Here's the drawing with two shaded views (mm, measured from the low corner). I have some questions. Give positions to 0.01 mm unless a question says otherwise; leave off trailing zeros. Loops run counter-clockwise (first coordinate to the right, second up) from the corner with the lowest first, then second, coordinate; pieces in that order, holes last. Notation, with made-up numbers: M -21,-32.75 L 3,-32.75 A32 cw 3,-1.75 Z; hole C 8,-35.5 d5. An arc over 180 degrees is marked long. Write item = value, one per line. Start each with the question number.
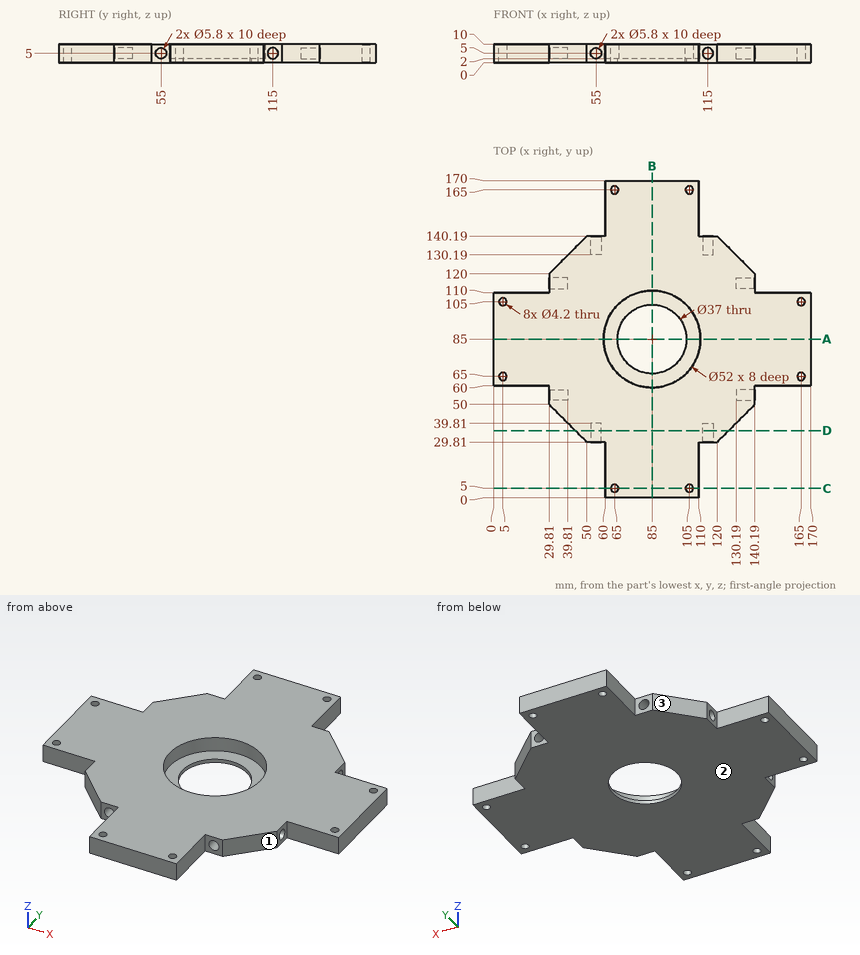
Q1. Will these pins go through, and if not, where does the flat tip stop? pin 1 (1.7 mm diameter, centred on y = 55.5, z = 6, fed in from -X); pin 2 (5 mm diameter, centred on x = 115, z = 5, fed in from +Y); pin 3 (2 mm diameter, centred on y = 19.5, z = 5.5, fed in from +X).
Q2. If we section it at A-A, the plane y = 85: List the corners of the cut face in (x, z) for me.
Q3. If we section it at C-C, the plane y = 5: List the corners of the cut face in (x, z) for me, then the cut area to 3 significant figures.
Q4. If I drill on line 1 along X through (y, z) = (165, 3); line 2 along X through (y, z) = (33.5, 5); line 3 along X through (y, z) = (104, 5.5), over which ranges is the centre line in solid material (lowest first)?
Q5. We'd pull the mould along Y, two halves only. Please class the marked faces 1, 2 and 3: pulls with the +Y half, pulls with the -Y half, needs draft (parallel to the pull), parting line crosses it, or undercut.
Q6. If we section it at D-D, the plane y = 36: List the corners of the cut face in (x, z) for me.
Resolved:
q1.pin_1 = 39.81
q1.pin_2 = 130.19
q1.pin_3 = 110
q2.outline = M 0,0 L 66.5,0 L 66.5,2 L 59,2 L 59,10 L 0,10 Z; M 103.5,0 L 170,0 L 170,10 L 111,10 L 111,2 L 103.5,2 Z
q3.outline = M 60,0 L 62.9,0 L 62.9,10 L 60,10 Z; M 67.1,0 L 102.9,0 L 102.9,10 L 67.1,10 Z; M 107.1,0 L 110,0 L 110,10 L 107.1,10 Z
q3.area = 416 mm²
q4.line_1 = 60 to 62.9, 67.1 to 102.9, 107.1 to 110
q4.line_2 = 46.31 to 52.1, 57.9 to 112.1, 117.9 to 123.69
q4.line_3 = 0 to 3.15, 6.85 to 67.25, 102.75 to 163.15, 166.85 to 170
q5.face_1 = pulls with the -Y half
q5.face_2 = needs draft
q5.face_3 = pulls with the +Y half
q6.outline = M 43.81,0 L 126.19,0 L 126.19,10 L 43.81,10 Z; hole C 55,5 d5.8; hole C 115,5 d5.8
